Here's how the part is built. I have some questions about the finished solid (model axes, mm). Round coordinates to 2 decimals unless told otherwise and drop trailing zeros. Write each loop counter-clockwise with the first axis right and the second up, starting at its lowest first coordinate (ties: lowest second). Pieces come first, ordered by that corner, then holes. Notation, with made-up numbers: (59.5, 10.5) -> (97.5, 10.5) arc R23 ccw to (97.5, 36.5) -> close; hole circle Ø7 at (44.25, 9.25). An arc over 180 degrees is marked (long way). Answer in a Markdown table with one row per item. Add a question column.
Solid Edge part; units mm, degrees
sketch "Sketch1" plane through (0, 0, 0) normal (0, 0, 1) x (1, 0, 0)
  line L0 (-44.7158, 62.7158) -> (-24.7158, 62.7158)
  line L1 (-24.7158, 62.7158) -> (-24.7158, -27.2842)
  line L2 (-24.7158, -27.2842) -> (-44.7158, -27.2842)
  line L3 (-44.7158, -27.2842) -> (-44.7158, 62.7158)
extrude "Protrusion1" add sketch "Sketch1" along normal blind 20
hole "Hole_1" at (-37.2158, -12.6892, 20) direction (0, 0, -1) diameter 6.5 end up to next
hole "Hole1" at (-37.2158, 48.1208, 20) direction (0, 0, -1) diameter 6.5 end up to next
properties material "Aluminum, 6061-T6"
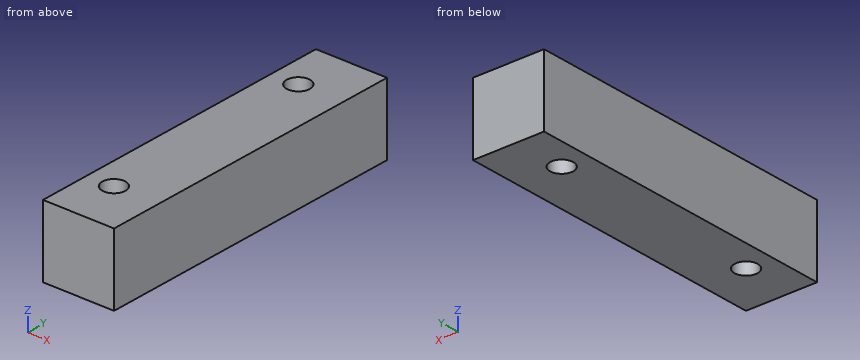
Item 1: If we section it at C-C on z = 13.5: Please give me the cut outline in (x, y).
Item 2: If we section it at D-D on y = -11.5: Please give me the cut outline in (x, z).
Item 3: I need wall thicknesses on line 1 along Y through (x, z) = (-35.25, 6); line 2 along Y through (x, z) = (-39, 10.25); line 3 along X through (y, z) = (47, 9). Which ranges of each line are inside material? Lowest first, please. Write a range as from..to.
Item 4: If we section it at A-A on y = 50: Please give me the cut outline in (x, z).
Item 5: If we section it at B-B on x = -39.5: Please give me the cut outline in (y, z).
Results list:
| question | item | result |
|---|---|---|
| 1 | outline | (-44.72, -27.28) -> (-24.72, -27.28) -> (-24.72, 62.72) -> (-44.72, 62.72) -> close; hole circle Ø6.5 at (-37.22, -12.69); hole circle Ø6.5 at (-37.22, 48.12) |
| 2 | outline | (-44.72, 0) -> (-40.24, 0) -> (-40.24, 20) -> (-44.72, 20) -> close; (-34.19, 0) -> (-24.72, 0) -> (-24.72, 20) -> (-34.19, 20) -> close |
| 3 | line 1 | -27.28..-15.28, -10.1..45.53, 50.71..62.72 |
| 3 | line 2 | -27.28..-15.41, -9.97..45.4, 50.84..62.72 |
| 3 | line 3 | -44.72..-40.27, -34.17..-24.72 |
| 4 | outline | (-44.72, 0) -> (-39.87, 0) -> (-39.87, 20) -> (-44.72, 20) -> close; (-34.56, 0) -> (-24.72, 0) -> (-24.72, 20) -> (-34.56, 20) -> close |
| 5 | outline | (-27.28, 0) -> (-15, 0) -> (-15, 20) -> (-27.28, 20) -> close; (-10.38, 0) -> (45.81, 0) -> (45.81, 20) -> (-10.38, 20) -> close; (50.43, 0) -> (62.72, 0) -> (62.72, 20) -> (50.43, 20) -> close |
